Could you check a few things on this model? Use its own coordinates, in mm. Give positions to 0.01 mm unless a question says otherwise; leave off trailing zeros. Write each loop counter-clockwise with the first axis right and the second up, starting at its lowest first coordinate (ties: lowest second). Pieces come first, ordered by that corner, then holes. Notation, with made-up numbers: M -10,6 L 46,6 A24 cw 46,32 Z; hole C 78.5,57.25 d10. An arc over 180 degrees is marked long. One line per item, written item: value.
```python
from build123d import *

# Parameters (mm, degrees)
SKETCH1_R           = 2.2
BOSS_EXTRUDE1_DEPTH = 6.35
FILLET1_R           = 1


with BuildPart() as part:
    # Sketch1 → Boss-Extrude1 (new body)
    with BuildSketch(Plane(origin=(0, 0, 0), x_dir=(0, 0, -1), z_dir=(1, 0, 0))):
        with BuildLine():
            Line((0, 6), (101.6, 6))
            ThreePointArc((101.6, 6), (107.6, 0), (101.6, -6))
            Line((101.6, -6), (0, -6))
            ThreePointArc((0, -6), (-6, 0), (0, 6))
        make_face()
        Circle(SKETCH1_R, mode=Mode.SUBTRACT)
        with Locations((101.6, 0)):
            Circle(SKETCH1_R, mode=Mode.SUBTRACT)
    extrude(amount=BOSS_EXTRUDE1_DEPTH)

    # Fillet1
    fillet1_edges = [part.edges().sort_by_distance(p)[0] for p in [
        (6.35, 0, -107.6),
        (6.35, 6, -50.8),
        (6.35, 0, 6),
        (0, 6, -50.8),
        (0, 0, -107.6),
        (0, -6, -50.8),
        (0, 0, 6),
        (6.35, -6, -50.8),
    ]]
    fillet(fillet1_edges, radius=FILLET1_R)


solid = part.part
```
1) Please list where these lines run through material, in increasing order: L1, parallel to Y at x = 1.5, z = 0; L2, parallel to Z at x = 2.5, y = -1.5; L3, parallel to Z at x = 2.75, y = 1. Write a range as from..to.
Outcome:
L1: y = -6..-2.2, 2.2..6
L2: z = -107.41..-103.21, -99.99..-1.61, 1.61..5.81
L3: z = -107.52..-103.56, -99.64..-1.96, 1.96..5.92
2) If we section it at A-A, the plane y = 0: Write out the boundary of the cut face in (x, z), then the cut area to 3 significant figures.
Outcome:
outline: M 0,-106.6 A1 ccw 1,-107.6 L 5.35,-107.6 A1 ccw 6.35,-106.6 L 6.35,-103.8 L 0,-103.8 Z; M 0,-99.4 L 6.35,-99.4 L 6.35,-2.2 L 0,-2.2 Z; M 0,2.2 L 6.35,2.2 L 6.35,5 A1 ccw 5.35,6 L 1,6 A1 ccw 0,5 Z
area: 665 mm^2
3) We'd pull the mould along Y, two halves only. Please class faces 1 (the face through (3.1, 0.1, -107.6)), 2 (the face through (3.13, 0.66, -103.7)), 3 (the face through (3, -6, -52)): pulls with the +Y half, pulls with the -Y half, needs draft (parallel to the pull), parting line crosses it, or undercut.
Outcome:
face 1: parting line crosses it
face 2: undercut
face 3: pulls with the -Y half
4) If we section it at B-B, the plane x = 2: Write out the boundary of the cut face in (y, z).
Outcome:
outline: M -6,-101.6 A6 ccw 6,-101.6 L 6,0 A6 ccw -6,0 Z; hole C 0,-101.6 d4.4; hole C 0,0 d4.4
